from build123d import *

# Parameters (mm, degrees)
SKETCH_1_W          = 160
SKETCH_1_H          = 65
EXTRUDE_1_DEPTH     = 55
CUT_EXTRUDE_3_DEPTH = 60
SKETCH_6_W          = 17
SKETCH_6_H          = 25
CUT_EXTRUDE_4_DEPTH = 60
SKETCH_7_W          = 27
SKETCH_7_H          = 25
CUT_EXTRUDE_5_DEPTH = 1.5
SKETCH_9_R          = 11.25
CUT_EXTRUDE_6_DEPTH = 10
FILLET_3_R          = 5
CUT_EXTRUDE_7_DEPTH = 2.34
SKETCH_12_R         = 1.5
CUT_EXTRUDE_8_DEPTH = 4


with BuildPart() as part:
    # Эскиз1 → Бобышка-Вытянуть1 (new body)
    with BuildSketch(Plane(origin=(0, 0, 0), x_dir=(0, 0, -1), z_dir=(1, 0, 0))):
        Rectangle(SKETCH_1_W, SKETCH_1_H)
    extrude(amount=EXTRUDE_1_DEPTH)

    # Эскиз2 → Вырез-Вытянуть3 (cut)
    with BuildSketch(Plane.XZ.offset(32.5)):
        Polygon((5, -71), (10, -71), (13, -71), (13, -75), (14, -75), (14, -71), (17, -71), (17, -75), (37, -75), (37, -71), (40, -71), (40, -75), (41, -75), (41, -71), (44, -71), (50, -71), (50, 71), (44, 71), (41, 71), (41, 75), (40, 75), (40, 71), (37, 71), (37, 75), (17, 75), (17, 71), (14, 71), (14, 75), (13, 75), (13, 71), (10, 71), (5, 71), align=None)
    extrude(amount=-CUT_EXTRUDE_3_DEPTH, mode=Mode.SUBTRACT)

    # Эскиз6 → Вырез-Вытянуть4 (cut)
    with BuildSketch(Plane(origin=(0, 32.5, 0), x_dir=(1, 0, 0), z_dir=(0, 1, 0))):
        with Locations((31.5, -37.5)):
            Rectangle(SKETCH_6_W, SKETCH_6_H)
    extrude(amount=-CUT_EXTRUDE_4_DEPTH, mode=Mode.SUBTRACT)

    # Эскиз7 → Вырез-Вытянуть5 (cut)
    with BuildSketch(Plane.XZ.offset(-27.5)):
        with Locations((31.5, 37.5)):
            Rectangle(SKETCH_7_W, SKETCH_7_H)
    extrude(amount=-CUT_EXTRUDE_5_DEPTH, mode=Mode.SUBTRACT)

    # Эскиз9 → Вырез-Вытянуть6 (cut)
    with BuildSketch(Plane(origin=(55, 0, 0), x_dir=(0, 0, -1), z_dir=(1, 0, 0))):
        with Locations((-39.25, 0.6)):
            Circle(SKETCH_9_R)
        with Locations((19.503, 0.6)):
            Circle(SKETCH_9_R)
        with Locations((44.903, 0.6)):
            Circle(SKETCH_9_R)
        with Locations((-13.85, 0.6)):
            Circle(SKETCH_9_R)
    extrude(amount=-CUT_EXTRUDE_6_DEPTH, mode=Mode.SUBTRACT)

    # Скругление3
    fillet_3_edges = [part.edges().sort_by_distance(p)[0] for p in [
        (55, 0, -80),
        (55, 0, 80),
        (27.5, 32.5, -80),
        (27.5, 32.5, 80),
        (55, 32.5, 0),
    ]]
    fillet(fillet_3_edges, radius=FILLET_3_R)

    # Эскиз10 → Вырез-Вытянуть7 (cut)
    with BuildSketch(Plane.XZ.offset(32.5)):
        Polygon((51.558845727, 72.3), (53.117691454, 75), (51.558845727, 77.7), (48.441154273, 77.7), (46.882308546, 75), (48.441154273, 72.3), align=None)
        Polygon((6.558845727, 72.3), (8.117691454, 75), (6.558845727, 77.7), (3.441154273, 77.7), (1.882308546, 75), (3.441154273, 72.3), align=None)
        Polygon((8.117691454, -75), (6.558845727, -72.3), (3.441154273, -72.3), (1.882308546, -75), (3.441154273, -77.7), (6.558845727, -77.7), align=None)
        Polygon((51.558845727, -77.7), (53.117691454, -75), (51.558845727, -72.3), (48.441154273, -72.3), (46.882308546, -75), (48.441154273, -77.7), align=None)
    extrude(amount=-CUT_EXTRUDE_7_DEPTH, mode=Mode.SUBTRACT)

    # Эскиз12 → Вырез-Вытянуть8 (cut)
    with BuildSketch(Plane.XZ.offset(32.5)):
        with Locations(Location((50, 75, 0), (0, 0, 270))):
            Circle(SKETCH_12_R)
        with Locations(Location((50, -75, 0), (0, 0, 270))):
            Circle(SKETCH_12_R)
        with Locations(Location((5, -75, 0), (0, 0, 270))):
            Circle(SKETCH_12_R)
        with Locations(Location((5, 75, 0), (0, 0, 270))):
            Circle(SKETCH_12_R)
    extrude(amount=-CUT_EXTRUDE_8_DEPTH, mode=Mode.SUBTRACT)


solid = part.part
Model file for the job. Use its own axes, mm. A direction names the side the tool comes from. Give positions to 0.01 mm unless a question says otherwise; leave off trailing zeros. Order: outer loops, then holes, each group sorted by start corner. A loop starts at its lowest first (then second) coordinate and runs counter-clockwise, first axis right, second up. Notation, with made-up numbers: (34.5, -29) - (81.5, -29) arc R8 cw to (81.5, -18) - close; hole circle Ø1 at (45, 8). An arc over 180 degrees is marked (long way). Write item = value, one per line. Start each with the question number.
1. Probe line 1 along X through (y, z) = (-11, 60); line 2 along Z through (x, y) = (22, 12); line 3 along Z through (x, y) = (47, 22.5). List the from-to ranges inside material, lowest first.
2. Cut at A-A, the plane z = 13.85. List the corners of the cut face in (x, y), and give its area (3 significant figures).
3. Which spindle directions (+Z, -Z, +X, -X, +Y, -Y) get a long thin tool onto all of the face, cutting with end or side? Do faces 5 (the flat face through (5, -28.5, 75)), 6 (the cylindrical face through (53, -2, 79)), 7 (the flat face through (40, 31, 38)). Say none if no direction does.
4. Two-plate mould, pull along Z, no slides. Class faces 1 (the flat face through (51.3, -30.16, 73.8)), 2 (the cylindrical face through (25.35, 31.07, -78.5)), 3 (the flat face through (6.3, -30.16, 73.8)), 4 (the flat face through (25, -3, 80)): pulls with the +Z half, pulls with the -Z half, needs draft (parallel to the pull), parting line crosses it, or undercut.
5. Cut at B-B, the plane x = 11. List the corners of the cut face in (y, z).
6. Drop flat-ended pins along their axis: P1, Ø1.6, axis at y = 28.5, z = 38, coming from the +X side; P2, Ø4, axis at x = 5, z = 75, coming from the -Y side; P3, Ø6, axis at x = 33.5, z = -48.5, coming from the -Y side. Give the stop position or say it passes through.
7. Cut at D-D, the plane z = -10.5. List the corners of the cut face in (x, y).
Taken from the geometry:
q1.line_1 = 0 to 5, 50 to 55
q1.line_2 = -80 to -75, 75 to 80
q1.line_3 = -80 to -71, 71 to 80
q2.outline = (0, -32.5) - (5, -32.5) - (5, 27.5) - (50, 27.5) - (50, 11.85) - (55, 11.85) - (55, 27.5) arc R5 ccw to (50, 32.5) - (0, 32.5) - close; (50, -32.5) - (55, -32.5) - (55, -10.65) - (50, -10.65) - close
q2.area = 757 mm²
q3.face_5 = -Y
q3.face_6 = +Z, +X, +Y, -Y
q3.face_7 = +Y, -Y
q4.face_1 = undercut
q4.face_2 = pulls with the -Z half
q4.face_3 = undercut
q4.face_4 = pulls with the +Z half
q5.outline = (-32.5, -80) - (27.5, -80) arc R5 ccw to (32.5, -75) - (32.5, 75) arc R5 ccw to (27.5, 80) - (-32.5, 80) - (-32.5, 71) - (27.5, 71) - (27.5, -71) - (-32.5, -71) - close
q6.P1 = 55
q6.P2 = -30.16
q6.P3 = 27.5
q7.outline = (0, -32.5) - (5, -32.5) - (5, 27.5) - (50, 27.5) - (50, 7.35) - (55, 7.35) - (55, 27.5) arc R5 ccw to (50, 32.5) - (0, 32.5) - close; (50, -32.5) - (55, -32.5) - (55, -6.15) - (50, -6.15) - close
